```python
from build123d import *

# Parameters (mm, degrees)
SKETCH_1_W                  = 42
SKETCH_1_H                  = 70
SKETCH_1_R                  = 3.815643184
EXTRUDE_1_DEPTH             = 10
SKETCH_2_R                  = 5
SKETCH_2_R_2                = 2.5
EXTRUDE_2_DEPTH             = 10
MIRROR_23_COPY_1_SKETCH_R   = 5
MIRROR_23_COPY_1_SKETCH_R_2 = 2.5
MIRROR_23_COPY_1_DEPTH      = 10
SKETCH_3_R                  = 3
CUT_EXTRUDE_1_DEPTH         = 5
SKETCH_4_R                  = 1.5
CUT_EXTRUDE_2_DEPTH         = 151.99366476
EXTRUDE_3_DEPTH             = 11


with BuildPart() as part:
    # Sketch 1 → Extrude 1 (new body)
    with BuildSketch(Plane(origin=(-10, 0, 0), x_dir=(0, 0, -1), z_dir=(1, 0, 0))):
        Rectangle(SKETCH_1_W, SKETCH_1_H)
        Circle(SKETCH_1_R, mode=Mode.SUBTRACT)
    extrude_1 = extrude(amount=EXTRUDE_1_DEPTH)


with BuildPart() as body_2:
    # Sketch 2 → Extrude 2 (new body)
    with BuildSketch(Plane.XY.offset(21)):
        with BuildLine():
            Line((0, 35), (99.693856574, 81.488008791))
            ThreePointArc((99.693856574, 81.488008791), (107.340240625, 81.821857129), (112.983117062, 76.651113539))
            Line((112.983117062, 76.651113539), (118.819711203, 64.134497011))
            ThreePointArc((118.819711203, 64.134497011), (119.15355954, 56.488112961), (113.98281595, 50.845236523))
            Line((113.98281595, 50.845236523), (112.170200376, 50))
            Line((112.170200376, 50), (112.170200376, 0))
            Line((112.170200376, 0), (85.78027682, 0))
            Line((85.78027682, 0), (85.78027682, 49.303144229))
            ThreePointArc((85.78027682, 49.303144229), (81.153272904, 57.737058687), (71.554094203, 58.366222099))
            Line((71.554094203, 58.366222099), (0, 25))
            Line((0, 25), (0, 35))
        make_face()
        with Locations((100, 35)):
            Circle(SKETCH_2_R, mode=Mode.SUBTRACT)
        with Locations((108.27716468, 65.429340608)):
            Circle(SKETCH_2_R_2, mode=Mode.SUBTRACT)
    extrude_2 = extrude(amount=-EXTRUDE_2_DEPTH)


with BuildPart() as part_1:
    add(part.part)

    add(body_2.part)  # Mirror 5 merges body 2
    # Mirror 5: Extrude 2 across plane
    add(extrude_2.mirror(Plane.ZX))

    # Mirror 23: Extrude 1, Extrude 2 across plane
    add(extrude_1.mirror(Plane.XY))
    add(extrude_2.mirror(Plane.XY))

    # Mirror 23 copy 1 sketch → Mirror 23 copy 1 (add)
    with BuildSketch(Plane(origin=(0, 0, -21), x_dir=(1, 0, 0), z_dir=(0, 0, -1))):
        with BuildLine():
            Line((0, 35), (99.693856574, 81.488008791))
            ThreePointArc((99.693856574, 81.488008791), (107.340240625, 81.821857129), (112.983117062, 76.651113539))
            Line((112.983117062, 76.651113539), (118.819711203, 64.134497011))
            ThreePointArc((118.819711203, 64.134497011), (119.15355954, 56.488112961), (113.98281595, 50.845236523))
            Line((113.98281595, 50.845236523), (112.170200376, 50))
            Line((112.170200376, 50), (112.170200376, 0))
            Line((112.170200376, 0), (85.78027682, 0))
            Line((85.78027682, 0), (85.78027682, 49.303144229))
            ThreePointArc((85.78027682, 49.303144229), (81.153272904, 57.737058687), (71.554094203, 58.366222099))
            Line((71.554094203, 58.366222099), (0, 25))
            Line((0, 25), (0, 35))
        make_face()
        with Locations((100, 35)):
            Circle(MIRROR_23_COPY_1_SKETCH_R, mode=Mode.SUBTRACT)
        with Locations((108.27716468, 65.429340608)):
            Circle(MIRROR_23_COPY_1_SKETCH_R_2, mode=Mode.SUBTRACT)
    extrude(amount=-MIRROR_23_COPY_1_DEPTH)

    # Sketch 3 → Cut-Extrude 1 (cut)
    with BuildSketch(Plane(origin=(0, 0, 0), x_dir=(0, 0, -1), z_dir=(1, 0, 0))):
        with Locations((15.5, 15.5)):
            Circle(SKETCH_3_R)
        with Locations((15.5, -15.5)):
            Circle(SKETCH_3_R)
        with Locations((-15.5, -15.5)):
            Circle(SKETCH_3_R)
        with Locations((-15.5, 15.5)):
            Circle(SKETCH_3_R)
    extrude(amount=-CUT_EXTRUDE_1_DEPTH, mode=Mode.SUBTRACT)

    # Sketch 4 → Cut-Extrude 2 (cut, through all)
    with BuildSketch(Plane(origin=(-5, 0, 0), x_dir=(0, 0, -1), z_dir=(1, 0, 0))):
        with Locations((15.5, 15.5)):
            Circle(SKETCH_4_R)
        with Locations((-15.5, 15.5)):
            Circle(SKETCH_4_R)
        with Locations((-15.5, -15.5)):
            Circle(SKETCH_4_R)
        with Locations((15.5, -15.5)):
            Circle(SKETCH_4_R)
    extrude(amount=-CUT_EXTRUDE_2_DEPTH, mode=Mode.SUBTRACT)

    # Sketch 5 → Extrude 3 (add, symmetric)
    with BuildSketch(Plane.XY):
        Polygon((0, 35), (0, 25), (5, 27.331538291), (10, 39.663076582), align=None)
    extrude_3 = extrude(amount=EXTRUDE_3_DEPTH, both=True)

    # Mirror 24: Extrude 3 across plane
    add(extrude_3.mirror(Plane.ZX))


solid = part_1.part
```
Check sheet for the modelled part. Datum: model origin and axes. Units: mm. A direction names the side the tool comes from. Coordinates: 2 decimals unless noted, no trailing zeros. Order: outer loops, then holes, each group sorted by start corner. A loop starts at its lowest first (then second) coordinate and runs counter-clockwise, first axis right, second up. Notation, with made-up numbers: (22.5, 88.25) -> (81.5, 88.25) arc R22 cw to (81.5, 124.25) -> close; hole circle Ø5 at (41, -26). An arc over 180 degrees is marked (long way). Write item = value, one per line. Start each with the question number.
1) Cross-section at D-D (x = 108). Enter the section's corners in (y, z), then the cut area to 3 significant figures.
2) Material ranges on L1, parallel to Y at x = -1.85, z = -15.5; L2, parallel to Z at x = 104, y = 58.5; L3, parallel to Z at x = -7, y = -15, recorded low to high.
3) Access from +Z, -Z, +X, -X, +Y, -Y to the whole of each face (thin tool, end or side, straight path). Record for faces 4 (the flat face through (-5, 35, 0)), 5 (the cylindrical face through (81.27, 57.66, -16.07)), 6 (the cylindrical face through (107.237, -81.859, -16.07)), 7 (the flat face through (-5, -17, 14)), 8 (the flat face through (112.17, -1, 16)).
4) Cross-section at A-A (z = -9). Enter the section's corners in (x, y).
5) Mould release check, pull along Z, two halves, no side actions. Record for faces 1 (the flat face through (92, 0, 11)), 2 (the flat face through (89, 0, 21)), 3 (the flat face through (115.86, 70.48, -16.07)): +Z half, -Z half, draft (parallel to the pull), parting line (faces both ways), or undercut.
6) Go/stop test with flat-tipped pins: P1, Ø3, axis at x = 108.28, y = -65.43, coming from the +Z side; P2, Ø3, axis at y = 1, z = -15, coming from the +X side; P3, Ø3.5, axis at y = -15.5, z = 15.5, coming from the -X side; P4, Ø11, axis at x = -7, z = -9.5, coming from the -Y side. Record where each tip stops, or that it passes through.
7) Cross-section at B-B (y = 0). Enter the section's corners in (x, z), then the cut area to 3 significant figures.
8) Cross-section at C-C (x = 51.5). Enter the section's corners in (y, z).
Ans:
q1.outline = (-81.55, -21) -> (-67.91, -21) -> (-67.91, -11) -> (-81.55, -11) -> close; (-81.55, 11) -> (-67.91, 11) -> (-67.91, 21) -> (-81.55, 21) -> close; (-62.94, -21) -> (62.94, -21) -> (62.94, -11) -> (-62.94, -11) -> close; (-62.94, 11) -> (62.94, 11) -> (62.94, 21) -> (-62.94, 21) -> close; (67.91, -21) -> (81.55, -21) -> (81.55, -11) -> (67.91, -11) -> close; (67.91, 11) -> (81.55, 11) -> (81.55, 21) -> (67.91, 21) -> close
q1.area = 3,060 mm²
q2.L1 = -35 to -18.5, -12.5 to 12.5, 18.5 to 35
q2.L2 = -21 to -11, 11 to 21
q2.L3 = -21 to -16.91, -14.09 to 14.09, 16.91 to 21
q3.face_4 = +Z, -Z, -X, +Y
q3.face_5 = +Z, -Z
q3.face_6 = +Z, -Z, -Y
q3.face_7 = none
q3.face_8 = +Z, -Z, +X
q4.outline = (-10, -35) -> (0, -35) -> (10, -39.66) -> (5, -27.33) -> (0, -25) -> (0, 25) -> (5, 27.33) -> (10, 39.66) -> (0, 35) -> (-10, 35) -> close
q5.face_1 = undercut
q5.face_2 = +Z half
q5.face_3 = draft
q6.P1 = through
q6.P2 = 112.17
q6.P3 = -10
q6.P4 = -35
q7.outline = (-10, -21) -> (0, -21) -> (0, -3.82) -> (-10, -3.82) -> close; (-10, 3.82) -> (0, 3.82) -> (0, 21) -> (-10, 21) -> close; (85.78, -21) -> (112.17, -21) -> (112.17, -11) -> (85.78, -11) -> close; (85.78, 11) -> (112.17, 11) -> (112.17, 21) -> (85.78, 21) -> close
q7.area = 871 mm²
q8.outline = (-59.01, -21) -> (-49.01, -21) -> (-49.01, -11) -> (-59.01, -11) -> close; (-59.01, 11) -> (-49.01, 11) -> (-49.01, 21) -> (-59.01, 21) -> close; (49.01, -21) -> (59.01, -21) -> (59.01, -11) -> (49.01, -11) -> close; (49.01, 11) -> (59.01, 11) -> (59.01, 21) -> (49.01, 21) -> close
